from build123d import *

# Parameters (mm, degrees)
BOSS_EXTRUDE1_DEPTH = 600
CUT_EXTRUDE2_DEPTH  = 16
CUT_EXTRUDE3_REACH  = 826.099
SKETCH5_R           = 16
CUT_EXTRUDE4_DEPTH  = 4


with BuildPart() as part:
    # Sketch1 → Boss-Extrude1 (new, symmetric)
    with BuildSketch(Plane(origin=(0, 0, 0), x_dir=(0, 0, -1), z_dir=(1, 0, 0))):
        with BuildLine():
            Line((8, 0), (8, 496.686291501))
            Line((8, 496.686291501), (147.078210487, 635.764501988))
            ThreePointArc((147.078210487, 635.764501988), (147.078210487, 647.078210487), (135.764501988, 647.078210487))
            Line((135.764501988, 647.078210487), (-8, 503.313708499))
            Line((-8, 503.313708499), (-8, 0))
            Line((-8, 0), (8, 0))
        make_face()
    extrude(amount=BOSS_EXTRUDE1_DEPTH, both=True)

    # Sketch2 → Cut-Extrude2 (cut)
    with BuildSketch(Plane.XY.offset(8)):
        Polygon((-600, 503.313708499), (-500, 0), (-600, 0), align=None)
        Polygon((600, 503.313708499), (300, 0), (600, 0), align=None)
    extrude(amount=-CUT_EXTRUDE2_DEPTH, mode=Mode.SUBTRACT)

    # Cut-Extrude3: up to this face of the body (flat: up to its plane)
    cut_extrude3_end = Plane(part.part.faces().sort_by_distance((0, 566.225396744, -77.539105243))[0])
    # Sketch3 → Cut-Extrude3 (cut, up to the picked face)
    with BuildSketch(Plane(origin=(0, 255.656854249, 255.656854249), x_dir=(1, 0, 0), z_dir=(0, 0.7071067811865477, 0.7071067811865475)), mode=Mode.PRIVATE) as cut_extrude3_sk1:
        Polygon((600, 350.239682094), (477.997973515, 561.553390593), (600, 561.553390593), align=None)
    cut_extrude3_tool1 = split(extrude(cut_extrude3_sk1.sketch, amount=-CUT_EXTRUDE3_REACH, mode=Mode.PRIVATE), bisect_by=cut_extrude3_end, keep=Keep.BOTH, mode=Mode.PRIVATE)
    # Sketch3 → Cut-Extrude3 (cut, up to the picked face)
    with BuildSketch(Plane(origin=(0, 255.656854249, 255.656854249), x_dir=(1, 0, 0), z_dir=(0, 0.7071067811865477, 0.7071067811865475)), mode=Mode.PRIVATE) as cut_extrude3_sk2:
        Polygon((-600, 350.239682094), (-558.924776017, 561.553390593), (-600, 561.553390593), align=None)
    cut_extrude3_tool2 = split(extrude(cut_extrude3_sk2.sketch, amount=-CUT_EXTRUDE3_REACH, mode=Mode.PRIVATE), bisect_by=cut_extrude3_end, keep=Keep.BOTH, mode=Mode.PRIVATE)
    add(cut_extrude3_tool1.solids().sort_by(Axis((559.332658, 602.927946, -91.614237), (0, -0.7071067811865477, -0.7071067811865475)))[0], mode=Mode.SUBTRACT)
    add(cut_extrude3_tool2.solids().sort_by(Axis((-586.308259, 602.927946, -91.614237), (0, -0.7071067811865477, -0.7071067811865475)))[0], mode=Mode.SUBTRACT)

    # Sketch5 → Cut-Extrude4 (cut)
    with BuildSketch(Plane(origin=(0, 0, -8), x_dir=(-1, 0, 0), z_dir=(0, 0, -1))):
        with Locations((430.63716206, 333.578975831)):
            Circle(SKETCH5_R)
        with Locations((176.078720833, 333.578975831)):
            Circle(SKETCH5_R)
        with Locations((176.078720833, 79.020534604)):
            Circle(SKETCH5_R)
        with Locations((430.63716206, 79.020534604)):
            Circle(SKETCH5_R)
    extrude(amount=-CUT_EXTRUDE4_DEPTH, mode=Mode.SUBTRACT)


solid = part.part
Could you check a few things on this model? Use its own coordinates, in mm. A direction names the side the tool comes from. Coordinates: 2 decimals unless noted, no trailing zeros. Write each loop counter-clockwise with the first axis right and the second up, starting at its lowest first coordinate (ties: lowest second). Pieces come first, ordered by that corner, then holes. Notation, with made-up numbers: (62.5, -22) - (90.5, -22) arc R31 cw to (90.5, 14) - close; hole circle Ø2 at (13.25, 25.25). An arc over 180 degrees is marked (long way). Put each result on its own line as item: value. Start each with the question number.
Q1. I want a section at D-D on x = -515.5. Write out the boundary of the cut face in (y, z).
Q2. I want a section at B-B on z = -120.5. Write out the boundary of the cut face in (x, y), plus the area to 3 significant figures.
Q3. I want a section at A-A on x = 178. Write out the boundary of the cut face in (y, z), plus the area to 3 significant figures.
Q4. Please list where these lines run through material, in increasing order: L1, parallel to Z at x = -75.5, y = 470; L2, parallel to Y at x = -185.5, z = -85; L3, parallel to Y at x = -210, z = -58.
Q5. Which directions (+Z, -Z, +X, -X, +Y, -Y) give clear straight access to the entire face, cutting with the end or side of a thin tool? Please do faces 1 (the flat face through (7, 245, -8)), 2 (the flat face through (452.1, 255.18, 0.11)), 3 (the flat face through (-430, 334, -4)).
Q6. I want a section at C-C on y = 427. Write out the boundary of the cut face in (x, z).
Q7. I'm going to push flat-ended pins straight in: P1, Ø16, axis at x = -182.5, y = 85, coming from the -Z side; P2, Ø19, axis at x = -430.64, y = 333.58, coming from the -Z side; P3, Ø12, axis at x = 338, z = -49.5, coming from the +Y side. Where does each tip first touch, or does it pass through?
Q8. Thinking about a two-plate mould opening in Y: for faces 4 (the flat face through (7.095, 565.252, -76.566)), 5 (the flat face through (-430, 79, -4)), 6 (the flat face through (-579.75, 571.4, -71.24)), 7 (the flat face through (-176, 334, -4)), which applies, pulls with the +Y half, pulls with the -Y half, needs draft (parallel to the pull), parting line crosses it, or undercut?
Checks:
1. outline: (78.01, -8) - (496.69, -8) - (635.76, -147.08) arc R8 ccw to (647.08, -135.76) - (503.31, 8) - (78.01, 8) - close
2. outline: (-567.79, 609.19) - (504.32, 609.19) - (495.08, 631.81) - (-564.68, 631.81) - close
2. area: 24,100 mm²
3. outline: (0, -8) - (496.69, -8) - (635.76, -147.08) arc R8 ccw to (647.08, -135.76) - (503.31, 8) - (0, 8) - close
3. area: 11,300 mm²
4. L1: -8 to 8
4. L2: 573.69 to 596.31
4. L3: 546.69 to 569.31
5. face 1: -Z, +X, -X, -Y
5. face 2: +Z, -Z, +X, -Y
5. face 3: -Z
6. outline: (-584.84, -8) - (554.51, -8) - (554.51, 8) - (-584.84, 8) - close
7. P1: z = -8
7. P2: z = -4
7. P3: y = 566.81
8. face 4: pulls with the -Y half
8. face 5: undercut
8. face 6: pulls with the +Y half
8. face 7: undercut
